Can you work these out from the drawing? Everything is in mm from the part's minimum corner. Round coordinates to 2 decimals unless told otherwise and drop trailing zeros. Write each loop counter-clockwise with the first axis right and the second up, starting at its lowest first coordinate (ties: lowest second). Pieces come first, ordered by that corner, then holes. Notation, with made-up numbers: M 37.25,61 L 72.25,61 A34 cw 72.25,100 Z; hole C -15.75,-15 d2. An arc over 180 degrees is marked long. Use one line per item in the form item = value. Start each with the question number.
Q1. I want a section at C-C on z = 9.25. State how many separate pieces and enclosed holes the cut face has, and give its area (3 significant figures).
Q2. I'm going to push flat-ended pins straight in: pin 1 Ø1 at (x, z) = (533, 2) entering from +Y; pin 2 Ø1 at (y, z) = (342.5, 10.5) entering from +X (1 decimal); pin 3 Ø12.5 at (x, y) = (175, 487.08) entering from +Z; pin 4 Ø2 at (y, z) = (63.5, 2) entering from -X. Where does each tip first touch, or does it pass through?
Q3. I need wall thicknesses on line 1 along X through (y, z) = (256, 3.5) (1 decimal); line 2 along X through (y, z) = (80, 13); line 3 along X through (y, z) = (332, 9) (1 decimal). Which ranges of each line are inside material? Lowest first, please. Write a range as from..to.
Q4. I want a section at A-A on x = 300. List the corners of the cut face in (y, z) for me.
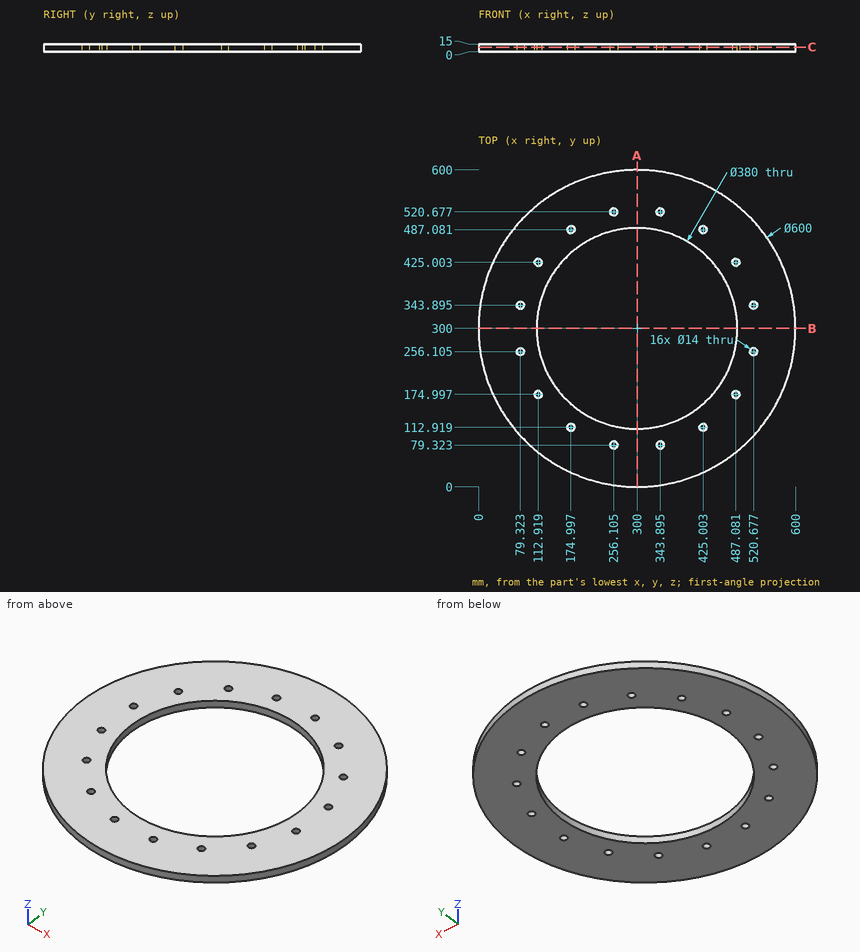
Reported:
q1.separate_pieces = 1
q1.enclosed_holes = 17
q1.area = 167,000 mm^2
q2.pin_1 = 489.59
q2.pin_2 = 597
q2.pin_3 = through
q2.pin_4 = 114.15
q3.line_1 = 3.2..72.3, 86.3..115.2, 484.8..513.7, 527.7..596.8
q3.line_2 = 96.04..249.14, 263.07..336.93, 350.86..503.96
q3.line_3 = 1.7..112.7, 487.3..598.3
q4.outline = M 0,0 L 110,0 L 110,15 L 0,15 Z; M 490,0 L 600,0 L 600,15 L 490,15 Z
